Verification items for this drawing (mm, ordinates from the low corner). A direction names the side the tool comes from. Round coordinates to 2 decimals unless told otherwise and drop trailing zeros. Order: outer loops, then holes, each group sorted by start corner. A loop starts at its lowest first (then second) coordinate and runs counter-clockwise, first axis right, second up. Notation, with made-up numbers: (34.5, 16.25) -> (57.5, 16.25) arc R37 cw to (57.5, 52.25) -> close; hole circle Ø4 at (78.5, -2.75). An arc over 180 degrees is marked (long way). Answer in a Markdown table with one row per item.
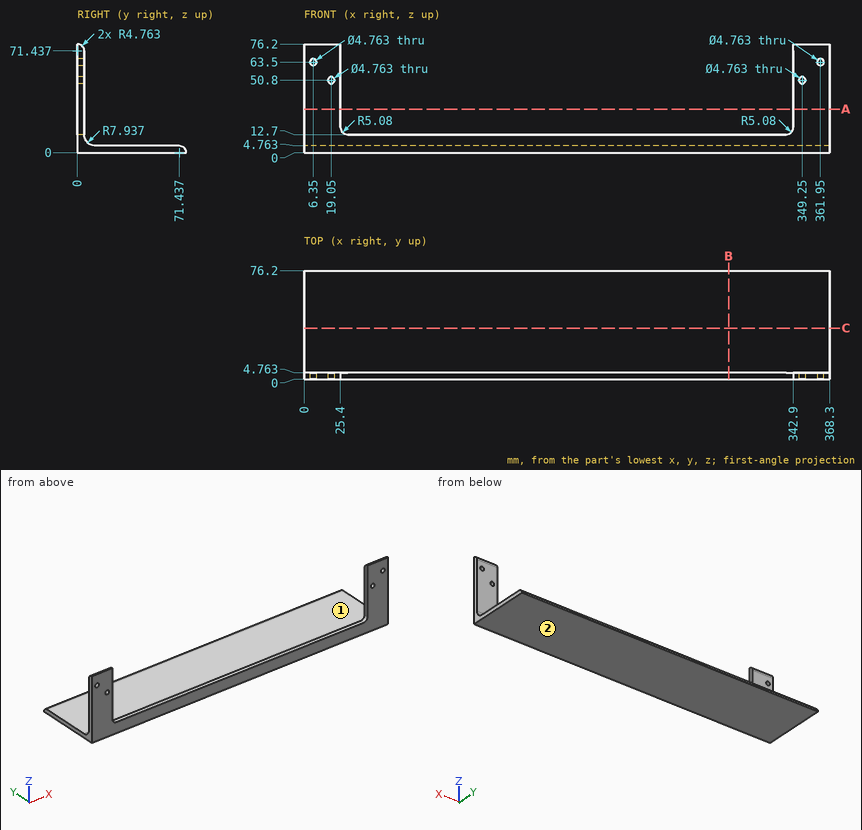
Item 1: Cross-section at B-B (x = 297.5). Record the boundary of the cut face in (y, z) (1 decimal).
Result sheet:
| item | result |
|---|---|
| outline | (0, 0) -> (76.2, 0) arc R4.8 ccw to (71.4, 4.8) -> (12.7, 4.8) arc R7.9 cw to (4.8, 12.7) -> (0, 12.7) -> close |
Item 2: Scan lines: line 1 (X direction, y = 3, z = 63); line 2 (Z direction, x = 179, y = 46.5). Record each from-to range of solid material in increasing order. Write a range as [from, to].
Result sheet:
| item | result |
|---|---|
| line 1 | x = [0, 4.02], [8.68, 25.4], [342.9, 359.62], [364.28, 368.3] |
| line 2 | z = [0, 4.76] |
Item 3: Depth check by flat-ended pin: P1, Ø8, axis at y = 9, z = 29.5, coming from the +X side; P2, Ø5, axis at x = 141.5, y = 3, coming from the +Z side; P3, Ø6, axis at x = 168, y = 63.5, coming from the +Z side; P4, Ø15, axis at x = 22.5, z = 47, coming from the +Y side. Enter the tip coordinate at first touch or a pass-through.
Result sheet:
| item | result |
|---|---|
| P1 | passes through |
| P2 | stops at z = 12.7 |
| P3 | stops at z = 4.76 |
| P4 | stops at y = 4.76 |
Item 4: Cross-section at A-A (z = 30.5). Record the boundary of the cut face in (x, y), and give its area (3 significant figures).
Result sheet:
| item | result |
|---|---|
| outline | (0, 0) -> (25.4, 0) -> (25.4, 4.76) -> (0, 4.76) -> close; (342.9, 0) -> (368.3, 0) -> (368.3, 4.76) -> (342.9, 4.76) -> close |
| area | 242 mm^2 |
Item 5: Cross-section at C-C (y = 36). Record the boundary of the cut face in (x, z), and give its area (3 significant figures).
Result sheet:
| item | result |
|---|---|
| outline | (0, 0) -> (368.3, 0) -> (368.3, 4.76) -> (0, 4.76) -> close |
| area | 1,750 mm^2 |
Item 6: Set-up check for the marked faces 1 and 2: record each of +Z, -Z, +X, -X, +Y, -Y from which the full face is reachable in a straight line by a thin tool's end or side.
Result sheet:
| item | result |
|---|---|
| face 1 | +Z, +X, -X, +Y |
| face 2 | -Z, +X, -X, +Y, -Y |
